Source: CAD feature listing. Evaluate the final solid. Frame: model axes, mm. A direction names the side the tool comes from. Give positions to 0.01 mm unless a question says otherwise; leave off trailing zeros. Write each loop counter-clockwise with the first axis right and the second up, starting at its lowest first coordinate (ties: lowest second). Pieces come first, ordered by that corner, then holes. Notation, with made-up numbers: (74, 74) -> (124, 74) arc R19 cw to (124, 111) -> close; hole circle Ø8 at (58, -6.75). An arc over 180 degrees is marked (long way). Answer as a JSON object with one key per item and string values. Group by question number.
Item 1: Section query B-B on z = 0. Return the cut outline in (x, y), plus the area to 3 significant figures.
Item 2: Pull-direction query (X, two-part tool) for faces 1 (the face through (5.848, -0.758, 0.01)), 2 (the face through (0.542, -0.814, -0.009)), 3 (the face through (0.56, 0, -0.56)); classes: pulls with the +X half, pulls with the -X half, needs draft (parallel to the pull), parting line crosses it, or undercut.
Item 3: Ray query, probe 1 along X at (y, z) = (0, 0); probe 2 along Z at (x, y) = (-3.25, 0.25); probe 3 along Z at (x, y) = (5.5, -0.55). Return the intervals inside material, ascending. Write a range as from..to.
Item 4: Access query for faces 4 (the face through (5.834, 0.742, 0.01)), 5 (the face through (-4, 0.75, 0)), 6 (the face through (-4, -0.75, 0)), 7 (the face through (-4, 0, 0.5)). Directions: +Z, -Z, +X, -X, +Y, -Y. A direction counts if a zero-diameter tool reaches every point of the face in a straight line with its end or side. Return the directions, or none.
Item 5: First-contact query: pin 1 Ø0.5 at (x, y) = (-6, 0.5) entering from -Z; pin 2 Ø0.8 at (x, y) = (4, -0.5) entering from -Z; pin 3 Ø0.8 at (x, y) = (-5, 0) entering from +Z. Flat tips, straight axial feed; report the tip coordinate or a pass-through.
Item 6: Section query A-A on x = 4.25. Return the cut outline in (y, z).
Item 7: Section query C-C on y = 0. Give the number of separate pieces and of enclosed holes in the cut face, plus the area to 3 significant figures.
Autodesk Inventor part; units mm, degrees
ref_plane "YZ Plane" through (0, 0, 0) normal (1, 0, 0) x (0, 1, 0)
ref_plane "XZ Plane" through (0, 0, 0) normal (0, 1, 0) x (-1, 0, 0)
ref_plane "XY Plane" through (0, 0, 0) normal (0, 0, 1) x (1, 0, 0)
sketch "Sketch1" plane through (0, 0, 0) normal (0, 0, 1) x (1, 0, 0)
  line L0 (-8.1593, 0.75) -> (1.3407, 0.75)
  line L1 (1.3407, -0.75) -> (-8.1593, -0.75)
  line L2 (-8.6593, -0.25) -> (-8.6593, 0.25)
  circle A0 centre (-6.6593, 0) radius 0.25
  circle A1 centre (2.3407, 0) radius 0.25
  line L3 (-11.6593, 0) -> (9.3407, 0)
  line L4 (1.3407, -0.75) -> (1.3407, -1.0115)
  line L5 (1.3407, 0.75) -> (1.3407, 0.9885)
  line L6 (-8.1593, 0.75) -> (-8.1593, 0.75)
  line L7 (-8.6593, 0.25) -> (-8.6593, 0.25)
  line L8 (-8.1593, -0.75) -> (-8.1593, -0.75)
  line L9 (-8.6593, -0.25) -> (-8.6593, -0.25)
  line L10 (1.3407, 0.9885) -> (5.3407, 0.9885)
  line L11 (6.3407, 0.4885) -> (6.3407, -0.5115)
  line L12 (1.3407, -1.0115) -> (5.3407, -1.0115)
  line L13 (5.3407, -1.0115) -> (6.3407, -0.5115)
  line L14 (5.3407, 0.9885) -> (6.3407, 0.4885)
  line L15 (-8.6593, 0.25) -> (-8.1593, 0.75)
  line L16 (-8.6593, -0.25) -> (-8.1593, -0.75)
  point P0 (0, 0)
  point P1 (-8.6593, 0.75)
  point P2 (-8.6593, -0.75)
  point P3 (6.3407, -1.0115)
  point P4 (6.3407, 0.9885)
  point P5 (-8.6593, 0)
  point P6 (6.3407, 0.9885)
  dimension "d2" = 0.5
  dimension "d4" = 0.5
  dimension "d34" = 9
  dimension "d36" = 1.5
  dimension "d37" = 2
  dimension "d38" = 2
  dimension "d39" = 8
  dimension "d40" = 5
  dimension "d56" = 1
  dimension "d57" = 0.5
  dimension "d58" = 1
  dimension "d59" = 0.5
  dimension "d60" = 0.5
  dimension "d61" = 0.5
  dimension "d62" = 0.5
  dimension "d63" = 0.5
extrude "Extrusion1" add sketch "Sketch1" along normal mid plane 1 contours L0 L5 L10 L14 L11 L3 A1 A0 L2 L15 | L3 A0 A1 L11 L13 L12 L4 L1 L16 L2
sketch "Sketch2" plane through (0, 0, 0.5) normal (0, 0, 1) x (1, 0, 0)
  circle A0 centre (2.3407, 0) radius 0.25
  circle A1 centre (-6.6593, 0) radius 0.25
  line L0 (1.3407, 0.75) -> (-8.1593, 0.75)
  line L1 (-8.6593, 0.25) -> (-8.6593, -0.25)
  line L2 (-8.1593, -0.75) -> (1.3407, -0.75)
  line L3 (1.3407, 0.75) -> (-8.1593, 0.75)
  line L4 (1.3407, 0.75) -> (1.3407, -0.75)
  line L5 (1.3407, -0.75) -> (1.3407, -1.0115)
  line L6 (1.3407, 0.9885) -> (1.3407, 0.75)
  line L7 (1.3407, -1.0115) -> (5.3407, -1.0115)
  line L8 (5.3407, -1.0115) -> (6.3407, -0.5115)
  line L9 (6.3407, -0.5115) -> (6.3407, 0.4885)
  line L10 (6.3407, 0.4885) -> (5.3407, 0.9885)
  line L11 (5.3407, 0.9885) -> (1.3407, 0.9885)
  line L12 (-8.1593, 0.75) -> (-8.6593, 0.25)
  line L13 (-8.6593, -0.25) -> (-8.1593, -0.75)
  point P0 (0, 0)
  point P1 (-8.6593, 0.75)
extrude "Extrusion2" add sketch "Sketch2" along normal blind 0.25 contours L6 L11 L10 L9 L8 L7 L5 L4
sketch "Sketch3" plane through (0, 0, -0.5) normal (0, 0, -1) x (-1, 0, 0)
  circle A0 centre (-2.3407, 0) radius 0.25
  circle A1 centre (6.6593, 0) radius 0.25
  line L0 (8.1593, 0.75) -> (-1.3407, 0.75)
  line L1 (-1.3407, -0.75) -> (8.1593, -0.75)
  line L2 (8.6593, -0.25) -> (8.6593, 0.25)
  line L3 (-0.3407, -0.75) -> (-0.3407, 0.75)
  line L4 (8.1593, -0.75) -> (-1.3407, -0.75)
  line L5 (-1.3407, 0.75) -> (-1.3407, -0.75)
  line L6 (-1.3407, 0.75) -> (-1.3407, 0.9885)
  line L7 (-1.3407, -1.0115) -> (-1.3407, -0.75)
  line L8 (8.1593, -0.75) -> (8.6593, -0.25)
  line L9 (8.6593, 0.25) -> (8.1593, 0.75)
  line L10 (-1.3407, 0.9885) -> (-5.3407, 0.9885)
  line L11 (-5.3407, 0.9885) -> (-6.3407, 0.4885)
  line L12 (-6.3407, 0.4885) -> (-6.3407, -0.5115)
  line L13 (-6.3407, -0.5115) -> (-5.3407, -1.0115)
  line L14 (-5.3407, -1.0115) -> (-1.3407, -1.0115)
  point P0 (0, 0)
  point P1 (8.6593, -0.75)
extrude "Extrusion3" add sketch "Sketch3" along normal blind 0.25 contours L5 L7 L14 L13 L12 L11 L10 L6
fillet "Fillet5" radius 5 4 edges at (1.3407, 0, 0.5) (1.3407, 0.75, 0) (1.3407, -0.75, 0) (1.3407, 0, -0.5)
sketch "Sketch10" plane through (0, 0, -0.75) normal (0, 0, -1) x (-1, 0, 0)
  circle A0 centre (-2.3407, 0) radius 0.25
  circle A1 centre (-2.3407, 0) radius 0.375
  circle A2 centre (-2.3407, 0) radius 0.5
  point P0 (0, 0)
  dimension "d48" = 0.75
  dimension "d49" = 1
extrude "Extrusion10" add sketch "Sketch10" along normal blind 0.15 contours A1
chamfer "Chamfer1" distance 0.1 angle 45 1 edges at (2.7157, 0, -0.75) measured on face at (4.4657, -0.0077, -0.75)
fillet "Fillet6" radius 0.25 1 edges at (3.3407, 0.9885, -0.75)
fillet "Fillet7" radius 0.25 3 edges at (3.3407, -1.0115, -0.75) (3.3407, -1.0115, 0.75) (3.3407, 0.9885, 0.75)
sketch "Sketch12" plane through (0, 0, -0.5) normal (0, 0, -1) x (-1, 0, 0)
  circle A0 centre (6.6593, 0) radius 0.25
  circle A1 centre (6.6593, 0) radius 0.625
  circle A2 centre (6.6593, 0) radius 0.375
  point P0 (0, 0)
  dimension "d66" = 1.25
  dimension "d67" = 0.75
extrude "Extrusion11" add sketch "Sketch12" along normal blind 0.25 contours A2
extrude "Extrusion12" add sketch "Sketch12" along normal blind 0.15 contours A1
fillet "Fillet8" radius 0.25 1 edges at (-6.2843, 0, -0.65)
fillet "Fillet9" radius 0.1 1 edges at (-6.0343, 0, -0.5)
sketch "Sketch14" plane through (6.3407, -0.5115, 0.75) normal (1, 0, 0) x (0, 0, -1)
  circle A0 centre (0.75, 0.5115) radius 0.25
  dimension "d77" = 0.5
extrude "Extrusion13" cut sketch "Sketch14" against normal blind 3
properties part number "Link_3"
Worked answers:
{
 "1": {"outline": "(-8.66, -0.25) -> (-8.16, -0.75) -> (-0.26, -0.75) arc R5 cw to (1.34, -1.01) -> (5.34, -1.01) -> (6.34, -0.51) -> (6.34, -0.25) -> (3.34, -0.25) -> (3.34, 0.25) -> (6.34, 0.25) -> (6.34, 0.49) -> (5.34, 0.99) -> (1.34, 0.99) arc R5 cw to (-0.19, 0.75) -> (-8.16, 0.75) -> (-8.66, 0.25) -> close; hole circle Ø0.5 at (-6.66, 0); hole circle Ø0.5 at (2.34, 0)", "area": "22.6 mm^2"},
 "2": {"face 1": "pulls with the +X half", "face 2": "pulls with the -X half", "face 3": "undercut"},
 "3": {"probe 1": "-8.66..-6.91, -6.41..2.09, 2.59..3.34", "probe 2": "-0.5..0.5", "probe 3": "-0.75..0.75"},
 "4": {"face 4": "+Z, -Z, +X, +Y", "face 5": "+Z, -Z, -X, +Y", "face 6": "+Z, -Z, -X, -Y", "face 7": "+Z, -X, +Y, -Y"},
 "5": {"pin 1": "z = -0.65", "pin 2": "z = -0.75", "pin 3": "z = 0.5"},
 "6": {"outline": "(-1.01, -0.5) arc R0.25 ccw to (-0.76, -0.75) -> (0.74, -0.75) arc R0.25 ccw to (0.99, -0.5) -> (0.99, 0.5) arc R0.25 ccw to (0.74, 0.75) -> (-0.76, 0.75) arc R0.25 ccw to (-1.01, 0.5) -> close; hole circle Ø0.5 at (0, 0)"},
 "7": {"separate pieces": "3", "enclosed holes": "0", "area": "15.2 mm^2"}
}
